```python
from build123d import *

# Parameters (mm, degrees)
F0_W          = 152.3185074329
F0_H          = 86.9983956218
F0_W_2        = 139.1974389553
F0_H_2        = 73.8773271441
F1_DEPTH      = 63.5
F2_W          = 61.6119801998
F2_H          = 38.222245872
F3_DEPTH      = 50.8
F3_DEPTH_BACK = 50.8
F4_R          = 9.10092064
F5_DEPTH      = 101.6
F5_DEPTH_BACK = 101.6


with BuildPart() as f1:
    # F0 (on Top) → F1 (new body)
    with BuildSketch(Plane.XY):
        Rectangle(F0_W, F0_H)
        Rectangle(F0_W_2, F0_H_2, mode=Mode.SUBTRACT)
    extrude(amount=F1_DEPTH)

    # F2 (on Front) → F3 (cut, two sides)
    with BuildSketch(Plane.XZ) as f3_sk:
        with Locations((0, 56.0497865081)):
            Rectangle(F2_W, F2_H)
    extrude(amount=F3_DEPTH, mode=Mode.SUBTRACT)
    extrude(f3_sk.sketch, amount=-F3_DEPTH_BACK, mode=Mode.SUBTRACT)

    # F4 (on Right) → F5 (cut, two sides)
    with BuildSketch(Plane.YZ) as f5_sk:
        with Locations((0, 34.656740725)):
            Circle(F4_R)
    extrude(amount=-F5_DEPTH, mode=Mode.SUBTRACT)
    extrude(f5_sk.sketch, amount=F5_DEPTH_BACK, mode=Mode.SUBTRACT)


solid = f1.part
```
Input: part model. Units: mm. Frame: model coordinates. A direction names the side the tool comes from. Give positions to 0.01 mm unless a question says otherwise; leave off trailing zeros. Order: outer loops, then holes, each group sorted by start corner. A loop starts at its lowest first (then second) coordinate and runs counter-clockwise, first axis right, second up. Notation, with made-up numbers: (28.5, 3) - (45.5, 3) arc R28 ccw to (45.5, 38) - close; hole circle Ø8 at (4.25, -1). An arc over 180 degrees is marked (long way). One line per item, written item: value.
1. Cut plane D-D, the plane y = 25.5. Output: boundary loops of the cut face in (x, z), and give its area (3 significant figures).
Determined:
outline: (-76.16, 0) - (-69.6, 0) - (-69.6, 63.5) - (-76.16, 63.5) - close; (69.6, 0) - (76.16, 0) - (76.16, 63.5) - (69.6, 63.5) - close
area: 833 mm2
2. Pin query (flat end, axial travel): pin 1 Ø5 at (x, y) = (-6, 42) entering from +Z. Return the tip coordinate at first contact, or that it passes through.
Determined:
pin 1: z = 36.94
3. Reachability of faces 1 (the face through (-69.599, -1, 24)), 2 (the face through (-1, 43.499, 31)), 3 (the face through (30.806, 40, 50)) from +Z, -Z, +X, -X, +Y, -Y: full face, straight path, thin tool, end or side. Return the list, or none.
Determined:
face 1: +Z, -Z
face 2: +Z, -Z, +X, -X, +Y
face 3: +Z, +Y, -Y
4. Cut plane B-B, the plane y = 0. Output: boundary loops of the cut face in (x, z), and give its area (3 significant figures).
Determined:
outline: (-76.16, 0) - (-69.6, 0) - (-69.6, 25.56) - (-76.16, 25.56) - close; (-76.16, 43.76) - (-69.6, 43.76) - (-69.6, 63.5) - (-76.16, 63.5) - close; (69.6, 0) - (76.16, 0) - (76.16, 25.56) - (69.6, 25.56) - close; (69.6, 43.76) - (76.16, 43.76) - (76.16, 63.5) - (69.6, 63.5) - close
area: 594 mm2
5. Cut plane A-A, the plane x = -38.5. Output: boundary loops of the cut face in (y, z).
Determined:
outline: (-43.5, 0) - (-36.94, 0) - (-36.94, 63.5) - (-43.5, 63.5) - close; (36.94, 0) - (43.5, 0) - (43.5, 63.5) - (36.94, 63.5) - close
6. Cut plane C-C, the plane z = 7. Output: boundary loops of the cut face in (x, y).
Determined:
outline: (-76.16, -43.5) - (76.16, -43.5) - (76.16, 43.5) - (-76.16, 43.5) - close; hole (-69.6, -36.94) - (69.6, -36.94) - (69.6, 36.94) - (-69.6, 36.94) - close
7. Draft query along X for faces 4 (the face through (-72.83, -1.18, 43.68)), 5 (the face through (-30.806, -40, 50)), 6 (the face through (76.159, -1, 24)). Return one class per face: released by +X, released by -X, zero draft, split by the parting line, or undercut.
Determined:
face 4: zero draft
face 5: undercut
face 6: released by +X
8. Line query: probe 1 along X at (y, z) = (-22, 15); probe 2 along Y at (x, z) = (25, 33); probe 3 along X at (y, z) = (39, 43.5). Output: solid intervals per line, ascending.
Determined:
probe 1: -76.16 to -69.6, 69.6 to 76.16
probe 2: -43.5 to -36.94, 36.94 to 43.5
probe 3: -76.16 to -30.81, 30.81 to 76.16
